Model file for the job. Use its own axes, mm. Give positions to 0.01 mm unless a question says otherwise; leave off trailing zeros. Loops run counter-clockwise (first coordinate to the right, second up) from the corner with the lowest first, then second, coordinate; pieces in that order, holes last. Notation, with made-up numbers: M 56.25,64.25 L 63.25,64.25 A22 cw 63.25,94.25 Z; hole C 8,31 d6. An arc over 180 degrees is marked long. Answer in a Markdown table with one row per item.
Autodesk Inventor part; units mm, degrees
ref_plane "YZ Plane" through (0, 0, 0) normal (1, 0, 0) x (0, 1, 0)
ref_plane "XZ Plane" through (0, 0, 0) normal (0, 1, 0) x (-1, 0, 0)
ref_plane "XY Plane" through (0, 0, 0) normal (0, 0, 1) x (1, 0, 0)
sketch "Sketch1" plane through (0, 0, 0) normal (0, 0, 1) x (1, 0, 0)
  line L0 (467.8685, 107.8942) -> (0, 196.85)
  line L1 (0, 0) -> (467.8685, 0)
  line L2 (0, 196.85) -> (0, 0)
  line L3 (467.8685, 107.8942) -> (467.8685, 0)
  line L4 (467.8685, 0) -> (468.4718, 0)
  line L5 (468.4718, 0) -> (468.4718, 107.7795)
  line L6 (468.4718, 107.7795) -> (467.8685, 107.8942)
  circle A0 centre (295.5085, 133.0828) radius 1.5875
  circle A1 centre (432.753, 107.0054) radius 1.5875
  circle A2 centre (364.1308, 120.0441) radius 1.5875
  circle A3 centre (226.8862, 146.1214) radius 1.5875
  line L7 (443.6664, 113.4153) -> (440.703, 97.8194) construction
  line L8 (443.6664, 113.4153) -> (219.0844, 156.0873) construction
  line L9 (216.1211, 140.4914) -> (219.0844, 156.0873) construction
  line L10 (440.703, 97.8194) -> (216.1211, 140.4914) construction
  circle A4 centre (230.3468, 7.5406) radius 1.5875
  circle A5 centre (436.7218, 7.5406) radius 1.5875
  circle A6 centre (23.9718, 7.5406) radius 1.5875
  line L11 (446.2468, 15.0813) -> (446.2468, -0.7937) construction
  line L12 (446.2468, 15.0813) -> (14.4468, 15.0813) construction
  line L13 (14.4468, -0.7937) -> (14.4468, 15.0813) construction
  line L14 (446.2468, -0.7937) -> (14.4468, -0.7937) construction
  circle A7 centre (4.3656, 95.25) radius 1.5875
  circle A8 centre (4.3656, 177.8) radius 1.5875
  circle A9 centre (4.3656, 12.7) radius 1.5875
  line L15 (-3.9687, 190.5) -> (11.9063, 190.5) construction
  line L16 (-3.9687, 190.5) -> (-3.9687, 0) construction
  line L17 (11.9063, 0) -> (-3.9687, 0) construction
  line L18 (11.9063, 190.5) -> (11.9063, 0) construction
  circle A10 centre (464.1061, 8.7313) radius 1.5875
  circle A11 centre (464.1061, 91.2812) radius 1.5875
  line L19 (456.5655, -0.7937) -> (471.6468, -0.7937) construction
  line L20 (456.5655, -0.7937) -> (456.5655, 100.8062) construction
  line L21 (471.6468, 100.8062) -> (456.5655, 100.8062) construction
  line L22 (471.6468, -0.7937) -> (471.6468, 100.8062) construction
  circle A12 centre (71.5968, 99.6156) radius 1.5875
  line L23 (81.1218, 107.95) -> (81.1218, 92.075) construction
  line L24 (81.1218, 107.95) -> (62.0718, 107.95) construction
  line L25 (62.0718, 92.075) -> (62.0718, 107.95) construction
  line L26 (81.1218, 92.075) -> (62.0718, 92.075) construction
  circle A13 centre (243.0468, 99.6156) radius 1.5875
  line L27 (252.5718, 107.95) -> (252.5718, 92.075) construction
  line L28 (252.5718, 107.95) -> (233.5218, 107.95) construction
  line L29 (233.5218, 92.075) -> (233.5218, 107.95) construction
  line L30 (252.5718, 92.075) -> (233.5218, 92.075) construction
  circle A14 centre (158.75, 154.8401) radius 1.5875
  line L31 (146.05, 145.3151) -> (146.05, 158.0151) construction
  line L32 (146.05, 145.3151) -> (171.45, 145.3151) construction
  line L33 (171.45, 158.0151) -> (171.45, 145.3151) construction
  line L34 (146.05, 158.0151) -> (171.45, 158.0151) construction
extrude "Extrusion1" add sketch "Sketch1" along normal blind 3.175
properties part number "Hopper Front" material "Polycarbonate, Clear"
(1) Saw through at B-B, the plane x = 347.5. Give the cut face in (y, z) (3 decimals), and give its area (3 significant figures).
Established:
| item | result |
|---|---|
| outline | M 0,0 L 130.78,0 L 130.78,3.175 L 0,3.175 Z |
| area | 415 mm2 |
(2) Wall check: L1, parallel to X at y = 95.25, z = 2.5; L2, parallel to Y at x = 242, z = 1.45; L3, parallel to Y at x = 194, z = 1.7. Give the ranges that are in metal, low to high.
Established:
| item | result |
|---|---|
| L1 | x = 0 to 2.78, 5.95 to 468.47 |
| L2 | y = 0 to 98.42, 100.81 to 150.84 |
| L3 | y = 0 to 159.96 |
(3) Saw through at C-C, the plane x = 193. Give the cut face in (y, z) (3 decimals), and give its area (3 significant figures).
Established:
| item | result |
|---|---|
| outline | M 0,0 L 160.155,0 L 160.155,3.175 L 0,3.175 Z |
| area | 508 mm2 |
(4) Saw through at A-A, the plane z = 1.3. Count the separate pieces of the cut face and the enclosed holes in it, and give its area (3 significant figures).
Established:
| item | result |
|---|---|
| separate pieces | 1 |
| enclosed holes | 15 |
| area | 71,200 mm2 |
